from build123d import *

# Parameters (mm, degrees)
F0_R      = 7.5
F1_DEPTH  = 150
F2_W      = 100
F2_H      = 60
F3_DEPTH  = 5
F4_DEPTH  = 5
F5_W      = 100
F5_H      = 60
F6_DEPTH  = 5
F7_R      = 5
F8_DEPTH  = 50
F9_R      = 5
F10_DEPTH = 10
F11_R     = 7.5
F12_DEPTH = 25
F14_DEPTH = 5


with BuildPart() as f1:
    # F0 (on Front) → F1 (new body, symmetric)
    with BuildSketch(Plane.XZ):
        Polygon((-12.5, 30), (-50, 30), (-50, -30), (50, -30), (50, 30), (12.5, 30), (12.5, 27), (47, 27), (47, -27), (-47, -27), (-47, 27), (-12.5, 27), align=None)
        Circle(F0_R)
    extrude(amount=F1_DEPTH, both=True)

    # F2 (on face) → F3 (join)
    with BuildSketch(Plane.XZ.offset(150)):
        Rectangle(F2_W, F2_H)
    extrude(amount=F3_DEPTH)

    # F2 (on face) → F4 (join)
    with BuildSketch(Plane.XZ.offset(150)):
        Rectangle(F2_W, F2_H)
    extrude(amount=F4_DEPTH)

    # F5 (on face) → F6 (join)
    with BuildSketch(Plane(origin=(0, 150, 0), x_dir=(-1, 0, 0), z_dir=(0, 1, 0))):
        Rectangle(F5_W, F5_H)
    extrude(amount=F6_DEPTH)

    # F7 (on face) → F8 (join)
    with BuildSketch(Plane(origin=(0, 0, -30), x_dir=(1, 0, 0), z_dir=(0, 0, -1))):
        with Locations((0, 30)):
            Circle(F7_R)
        with Locations((0, -30)):
            Circle(F7_R)
    extrude(amount=F8_DEPTH)

    # F9 (on face) → F10 (join)
    with BuildSketch(Plane(origin=(0, 0, -80), x_dir=(1, 0, 0), z_dir=(0, 0, -1))):
        with BuildLine():
            Line((18, 22.666667), (8, 36))
            ThreePointArc((8, 36), (0, 40), (-8, 36))
            Line((-8, 36), (-18, 22.666667))
            ThreePointArc((-18, 22.666667), (-19.486833, 19.828944), (-20, 16.666667))
            Line((-20, 16.666667), (-20, -16.666667))
            ThreePointArc((-20, -16.666667), (-19.486833, -19.828944), (-18, -22.666667))
            Line((-18, -22.666667), (-8, -36))
            ThreePointArc((-8, -36), (0, -40), (8, -36))
            Line((8, -36), (18, -22.666667))
            ThreePointArc((18, -22.666667), (19.486833, -19.828944), (20, -16.666667))
            Line((20, -16.666667), (20, 16.666667))
            ThreePointArc((20, 16.666667), (19.486833, 19.828944), (18, 22.666667))
        make_face()
        with Locations((0, 30)):
            Circle(F9_R, mode=Mode.SUBTRACT)
        with Locations((0, 30)):
            Circle(F9_R)
    extrude(amount=F10_DEPTH)

    # F11 (on face) → F12 (join)
    with BuildSketch(Plane(origin=(0, 0, -90), x_dir=(1, 0, 0), z_dir=(0, 0, -1))):
        with Locations((0, 30)):
            Circle(F11_R)
    extrude(amount=F12_DEPTH)

    # F13 (on face) → F14 (join)
    with BuildSketch(Plane(origin=(0, 0, -115), x_dir=(1, 0, 0), z_dir=(0, 0, -1))):
        with BuildLine():
            Line((-2.721043, 68.291105), (-7.440829, 30.940249))
            ThreePointArc((-7.440829, 30.940249), (0, 22.5), (7.440829, 30.940249))
            Line((7.440829, 30.940249), (2.721043, 68.291105))
            ThreePointArc((2.721043, 68.291105), (2.059421, 69.540617), (0.736823, 70.040372))
            Line((0.736823, 70.040372), (-0.736823, 70.040372))
            ThreePointArc((-0.736823, 70.040372), (-2.059421, 69.540617), (-2.721043, 68.291105))
        make_face()
    extrude(amount=-F14_DEPTH)


solid = f1.part
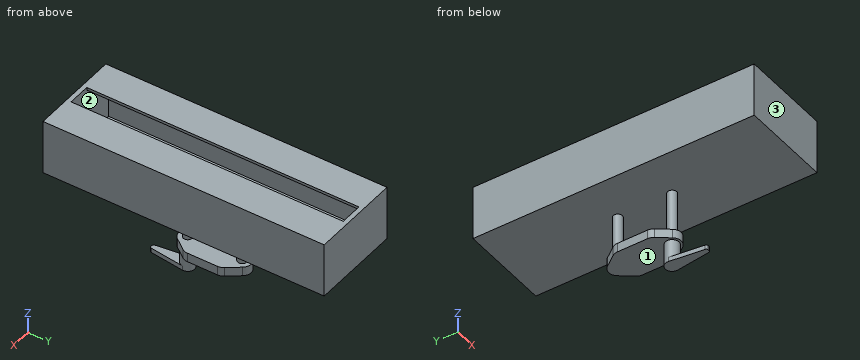
Build history of the part. All positions in model axes, mm. Face numbers are marked on the shaded views. Give positions to 0.01 mm unless a question says otherwise; leave off trailing zeros. Loops run counter-clockwise (first coordinate to the right, second up) from the corner with the lowest first, then second, coordinate; pieces in that order, holes last. Notation, with made-up numbers: (89, 31.25) -> (109, 31.25) arc R14 cw to (109, 49.25) -> close; hole circle Ø1 at (-33.5, 11.25). An arc over 180 degrees is marked (long way). Answer in a Markdown table with one row per item.
Item 1: Slice it at B-B on z = 21. Write the cut outline in (x, y).
Findings below:
| item | result |
|---|---|
| outline | (-50, -155) -> (50, -155) -> (50, 155) -> (-50, 155) -> close; hole (-47, -150) -> (47, -150) -> (47, 150) -> (-47, 150) -> close |
Item 2: Mould opens along Y. For the marked faces 1, 2 and 3 say: pulls with the +Y half, pulls with the -Y half, needs draft (parallel to the pull), parting line crosses it, or undercut.
Findings below:
| item | result |
|---|---|
| face 1 | needs draft |
| face 2 | undercut |
| face 3 | pulls with the -Y half |
Item 3: Slice it at A-A on y = 124.5. Write the cut outline in (x, z), plus the area to 3 significant figures.
Findings below:
| item | result |
|---|---|
| outline | (-50, -30) -> (50, -30) -> (50, 30) -> (12.5, 30) -> (12.5, 27) -> (47, 27) -> (47, -27) -> (-47, -27) -> (-47, 27) -> (-12.5, 27) -> (-12.5, 30) -> (-50, 30) -> close; circle Ø15 at (0, 0) |
| area | 1,030 mm² |
Item 4: Slice it at C-C on y = 11. Write the cut outline in (x, z), plus the area to 3 significant figures.
Findings below:
| item | result |
|---|---|
| outline | (-50, -30) -> (50, -30) -> (50, 30) -> (12.5, 30) -> (12.5, 27) -> (47, 27) -> (47, -27) -> (-47, -27) -> (-47, 27) -> (-12.5, 27) -> (-12.5, 30) -> (-50, 30) -> close; (-20, -90) -> (20, -90) -> (20, -80) -> (-20, -80) -> close; circle Ø15 at (0, 0) |
| area | 1,430 mm² |
Item 5: Flat gauge pins, fed straight in: P1, Ø8, axis at x = -24.5, y = -10.5, coming from the -Z side; P2, Ø8, axis at y = 7, z = -87, coming from the +X side; P3, Ø3, axis at x = -8, y = -38.5, coming from the +Z side. Where does each tip first touch, or does it go through?
Findings below:
| item | result |
|---|---|
| P1 | stops at z = -30 |
| P2 | stops at x = 20 |
| P3 | stops at z = 3.74 |
Item 6: Probe line 1 along X through (y, z) = (31, -22.5); line 2 along X through (y, z) = (80.5, -1); line 3 along Y through (x, z) = (33, -12). List the from-to ranges inside material, lowest first. Write a range as [from, to].
Findings below:
| item | result |
|---|---|
| line 1 | x = [-50, -47], [47, 50] |
| line 2 | x = [-50, -47], [-7.43, 7.43], [47, 50] |
| line 3 | y = [-155, -150], [150, 155] |
Item 7: Slice it at D-D on z = 0. Write the cut outline in (x, y), plus the area to 3 significant figures.
Findings below:
| item | result |
|---|---|
| outline | (-50, -155) -> (50, -155) -> (50, 155) -> (-50, 155) -> close; hole (-47, -150) -> (-7.5, -150) -> (-7.5, 150) -> (-47, 150) -> close; hole (7.5, -150) -> (47, -150) -> (47, 150) -> (7.5, 150) -> close |
| area | 7,300 mm² |
